from build123d import *

# Parameters (mm, degrees)
CROQUIS1_W              = 9.1
CROQUIS1_H              = 9.1
SALIENTE_EXTRUIR1_DEPTH = 55
CROQUIS2_R              = 1.95
CORTAR_EXTRUIR1_DEPTH   = 13
CROQUIS3_R              = 1.95
CORTAR_EXTRUIR2_DEPTH   = 10


with BuildPart() as part:
    # Croquis1 → Saliente-Extruir1 (new body)
    with BuildSketch(Plane(origin=(0, 0, 0), x_dir=(1, 0, 0), z_dir=(0, 1, 0))):
        with Locations((4.55, 4.55)):
            Rectangle(CROQUIS1_W, CROQUIS1_H)
    extrude(amount=SALIENTE_EXTRUIR1_DEPTH)

    # Croquis2 → Cortar-Extruir1 (cut)
    with BuildSketch(Plane(origin=(0, 55, 0), x_dir=(1, 0, 0), z_dir=(0, 1, 0))):
        with Locations((4.55, 4.55)):
            Circle(CROQUIS2_R)
    extrude(amount=-CORTAR_EXTRUIR1_DEPTH, mode=Mode.SUBTRACT)

    # Croquis3 → Cortar-Extruir2 (cut)
    with BuildSketch(Plane.XZ):
        with Locations((4.55, -4.55)):
            Circle(CROQUIS3_R)
    extrude(amount=-CORTAR_EXTRUIR2_DEPTH, mode=Mode.SUBTRACT)


solid = part.part
Geometry: final body of the model. Coordinates: model frame, mm. A direction names the side the tool comes from. Coordinates: 2 decimals unless noted, no trailing zeros. Loops run counter-clockwise (first coordinate to the right, second up) from the corner with the lowest first, then second, coordinate; pieces in that order, holes last. Notation, with made-up numbers: (56.25, 18) - (84.25, 18) arc R31 ccw to (84.25, 51) - close; hole circle Ø2 at (-12.75, 88). An arc over 180 degrees is marked (long way). One line per question, with ' | ' between items. Start each with the question number.
(1) Reachability of faces 4 (the flat face through (5, 10, -5)), 5 (the flat face through (2, 0, -5)), 6 (the cylindrical face through (2.6, 48.6, -4.6)) from +Z, -Z, +X, -X, +Y, -Y: full face, straight path, thin tool, end or side. Return the list, or none.
(2) First-contact query: pin 1 (3.5 mm diameter, centred on x = 4.55, z = -4.55, fed in from -Y). Flat tip, straight axial feed; report the tip coordinate or a pass-through.
(3) Cut plane C-C on x = 4.55. Output: boundary loops of the cut face in (y, z).
(4) Draft query along X for faces 1 (the cylindrical face through (2.6, 4.9, -4.5)), 2 (the flat face through (9.1, 27, -4)), 3 (the flat face through (4, 27, 0)). Return one class per face: +X half, -X half, draft (parallel to the pull), parting line (faces both ways), or undercut.
(5) Ray query, L1, parallel to X at y = 45, z = -4.55; L2, parallel to Z at x = 4.55, y = 46; L3, parallel to Y at x = 3.75, z = -3.5. Return the intervals inside material, ascending. Write a range as from..to.
(6) Cut plane B-B on z = -4.55. Output: boundary loops of the cut face in (x, y), and give its area (3 significant figures).
(7) Cut plane A-A on y = 50. Output: boundary loops of the cut face in (x, z).
Here are the results:
1) face 4: -Y | face 5: +Z, -Z, +X, -X, -Y | face 6: +Y
2) pin 1: y = 10
3) outline: (0, -9.1) - (55, -9.1) - (55, -6.5) - (42, -6.5) - (42, -2.6) - (55, -2.6) - (55, 0) - (0, 0) - (0, -2.6) - (10, -2.6) - (10, -6.5) - (0, -6.5) - close
4) face 1: undercut | face 2: +X half | face 3: draft
5) L1: 0..2.6, 6.5..9.1 | L2: -9.1..-6.5, -2.6..0 | L3: 10..42
6) outline: (0, 0) - (2.6, 0) - (2.6, 10) - (6.5, 10) - (6.5, 0) - (9.1, 0) - (9.1, 55) - (6.5, 55) - (6.5, 42) - (2.6, 42) - (2.6, 55) - (0, 55) - close | area: 411 mm²
7) outline: (0, -9.1) - (9.1, -9.1) - (9.1, 0) - (0, 0) - close; hole circle Ø3.9 at (4.55, -4.55)
